Source: CAD feature listing. Evaluate the final solid. Frame: model axes, mm. Face numbers are marked on the shaded views. Give positions to 0.01 mm unless a question says otherwise; leave off trailing zeros. Order: outer loops, then holes, each group sorted by start corner. A loop starts at its lowest first (then second) coordinate and runs counter-clockwise, first axis right, second up. Notation, with made-up numbers: (-38.75, 80) - (1.25, 80) arc R28 ccw to (1.25, 117) - close; hole circle Ø3 at (20.25, 33). An arc over 180 degrees is marked (long way). Write each question's results on one line, items separated by ' | '. Start each with the question number.
Item 1: Line query: line 1 along Y through (x, z) = (10.5, 10.5); line 2 along X through (y, z) = (-29, 0); line 3 along X through (y, z) = (-14, 9). Output: solid intervals per line, ascending.
Item 2: Contact query for flat-ended pins moving along their axis: pin 1 Ø6 at (x, z) = (8.5, -0.5) entering from -Y; pin 2 Ø3 at (x, y) = (11.5, -19.5) entering from -Z; pin 3 Ø5 at (y, z) = (-15, -4.5) entering from -X; pin 4 Ø2 at (y, z) = (-23.5, -10.5) entering from +X. Output: stop coordinate, or through.
Item 3: Section C-C on y = -24.5. Output: boundary loops of the cut face in (x, z).
Item 4: Section B-B on x = 0. State how many separate pieces and enclosed holes the cut face has, and give its area (4 significant figures).
Item 5: Section A-A on z = -13. Output: boundary loops of the cut face in (x, y).
Item 6: Section D-D on z = 0. Output: boundary loops of the cut face in (x, y), and give its area (3 significant figures).
Item 7: Mould query, pull axis X, two halves, no side actions, for the marked faces 1, 2 and 3. Classes: released by +X, released by -X, zero draft, split by the parting line, or undercut.
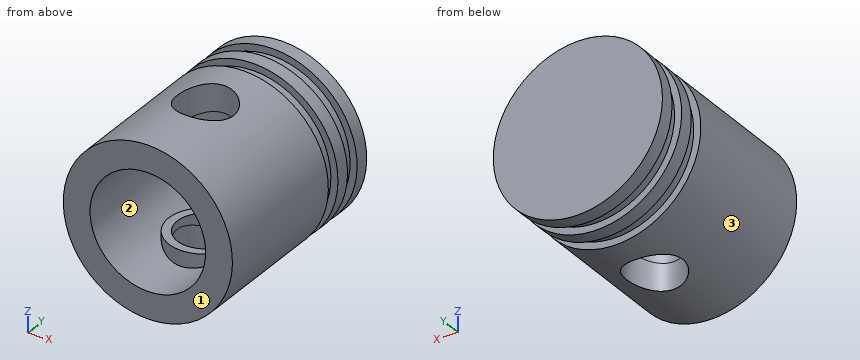
```python
from build123d import *

# Parameters (mm, degrees)
SKETCH1_R           = 15
BOSS_EXTRUDE1_DEPTH = 35
SKETCH2_W           = 1.25
SKETCH2_H           = 2.5
SKETCH4_R           = 5
CUT_EXTRUDE1_DEPTH  = 15
SKETCH5_R           = 10.25
CUT_EXTRUDE2_DEPTH  = 25
SKETCH6_R           = 6.5
SKETCH6_R_2         = 5
BOSS_EXTRUDE2_DEPTH = 12.5
SKETCH9_W           = 15
SKETCH9_H           = 15
CUT_EXTRUDE4_DEPTH  = 13


with BuildPart() as part:
    # Sketch1 → Boss-Extrude1 (new body)
    with BuildSketch(Plane(origin=(0, 0, 0), x_dir=(1, 0, 0), z_dir=(0, 1, 0))):
        with Locations(Location((0, 0, 0), (0, 0, 270))):
            Circle(SKETCH1_R)
    extrude(amount=-BOSS_EXTRUDE1_DEPTH)

    # Sketch2 → Cut-Revolve3 (revolve, cut)
    with BuildSketch(Plane.XY, mode=Mode.PRIVATE) as cut_revolve3_sk:
        with Locations((-14.375, -3.75)):
            Rectangle(SKETCH2_W, SKETCH2_H)
        with Locations((-14.375, -8.75)):
            Rectangle(SKETCH2_W, SKETCH2_H)
    revolve(cut_revolve3_sk.sketch.rotate(Axis((0, 0, 0), (0, 1, 0)), 90), axis=Axis((0, 0, 0), (0, 1, 0)), mode=Mode.SUBTRACT)

    # Sketch4 → Cut-Extrude1 (cut, symmetric)
    with BuildSketch(Plane.XY):
        with Locations(Location((0, -20, 0), (0, 0, 90))):
            Circle(SKETCH4_R)
    extrude(amount=CUT_EXTRUDE1_DEPTH, both=True, mode=Mode.SUBTRACT)

    # Sketch5 → Cut-Extrude2 (cut)
    with BuildSketch(Plane(origin=(0, -35, 0), x_dir=(-1, 0, 0), z_dir=(0, -1, 0))):
        with Locations(Location((0, 0, 0), (0, 0, 90))):
            Circle(SKETCH5_R)
    extrude(amount=-CUT_EXTRUDE2_DEPTH, mode=Mode.SUBTRACT)

    # Sketch6 → Boss-Extrude2 (add, symmetric)
    with BuildSketch(Plane.XY):
        with Locations(Location((0, -20, 0), (0, 0, 180))):
            Circle(SKETCH6_R)
        with Locations(Location((0, -20, 0), (0, 0, 90))):
            Circle(SKETCH6_R_2, mode=Mode.SUBTRACT)
    extrude(amount=BOSS_EXTRUDE2_DEPTH, both=True)

    # Sketch9 → Cut-Extrude4 (cut)
    with BuildSketch(Plane(origin=(6.5, 0, 0), x_dir=(0, 0, -1), z_dir=(1, 0, 0))):
        with Locations((0, -20.153875376)):
            Rectangle(SKETCH9_W, SKETCH9_H)
    extrude(amount=-CUT_EXTRUDE4_DEPTH, mode=Mode.SUBTRACT)


solid = part.part
```
Evaluation:
1) line 1: y = -35 to -10, -7.5 to -5, -2.5 to 0 | line 2: x = -15 to -10.25, 10.25 to 15 | line 3: x = -12 to -4.91, -2.5 to 2.5, 4.91 to 12
2) pin 1: stops at y = -35 | pin 2: stops at z = -11.18 | pin 3: stops at x = -14.87 | pin 4: stops at x = 11.61
3) outline: (-4.69, -9.11) arc R10.25 cw to (-4.69, 9.11) - (-4.69, 7.5) - (-2.18, 7.5) - (-2.18, 14.84) arc R15 ccw to (-2.18, -14.84) - (-2.18, -7.5) - (-4.69, -7.5) - close; (2.18, -14.84) arc R15 ccw to (2.18, 14.84) - (2.18, 7.5) - (4.69, 7.5) - (4.69, 9.11) arc R10.25 cw to (4.69, -9.11) - (4.69, -7.5) - (2.18, -7.5) - close
4) separate pieces: 3 | enclosed holes: 0 | area: 446.5 mm^2
5) outline: (-7.48, -35) - (7.48, -35) - (7.48, -10) - (4.48, -10) - (4.48, -7.5) - (7.48, -7.5) - (7.48, -5) - (4.48, -5) - (4.48, -2.5) - (7.48, -2.5) - (7.48, 0) - (-7.48, 0) - (-7.48, -2.5) - (-4.48, -2.5) - (-4.48, -5) - (-7.48, -5) - (-7.48, -7.5) - (-4.48, -7.5) - (-4.48, -10) - (-7.48, -10) - close; hole circle Ø10 at (0, -20)
6) outline: (-15, -35) - (-10.25, -35) - (-10.25, -10) - (10.25, -10) - (10.25, -35) - (15, -35) - (15, -10) - (13.75, -10) - (13.75, -7.5) - (15, -7.5) - (15, -5) - (13.75, -5) - (13.75, -2.5) - (15, -2.5) - (15, 0) - (-15, 0) - (-15, -2.5) - (-13.75, -2.5) - (-13.75, -5) - (-15, -5) - (-15, -7.5) - (-13.75, -7.5) - (-13.75, -10) - (-15, -10) - close | area: 525 mm^2
7) face 1: zero draft | face 2: undercut | face 3: split by the parting line
